```python
from build123d import *

# Parameters (mm, degrees)
F0_R     = 22.365
F1_DEPTH = 2
F2_R     = 2.5
F3_DEPTH = 45
F4_R     = 2


# Not quite as in the source:
# - a feature of the source that left no trace in its solid (it failed there, or was rolled back) is left out


with BuildPart() as f1:
    # F0 (on Top) → F1 (new body)
    with BuildSketch(Plane.XY):
        Polygon((26.865, -15.5105149818), (26.865, 15.5105149818), (0, 31.0210299636), (-26.865, 15.5105149818), (-26.865, -15.5105149818), (0, -31.0210299636), align=None)
        Circle(F0_R, mode=Mode.SUBTRACT)
        Circle(F0_R)
    extrude(amount=F1_DEPTH)

    # F2 (on face) → F3 (join)
    with BuildSketch(Plane.XY.offset(2)):
        with Locations((-14.5547939909, 0)):
            Circle(F2_R)
        with Locations((6.3876030045, 12.604821343)):
            Circle(F2_R)
        with Locations((6.8325, -11.8342371427)):
            Circle(F2_R)
    extrude(amount=F3_DEPTH)

    # F4
    f4_edges = [f1.edges().sort_by_distance(p)[0] for p in [
        (-17.054794, 0, 47),
        (4.3325, -11.834237, 47),
        (3.887603, 12.604821, 47),
    ]]
    fillet(f4_edges, radius=F4_R)


solid = f1.part
```
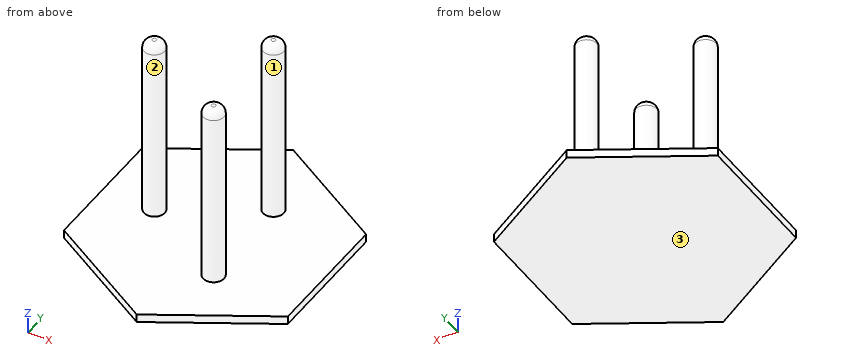
Geometry: final body of the model. Coordinates: model frame, mm. Face numbers are marked on the shaded views. Round coordinates to 2 decimals unless told otherwise and drop trailing zeros. Loops run counter-clockwise (first coordinate to the right, second up) from the corner with the lowest first, then second, coordinate; pieces in that order, holes last.
Item 1: Mould query, pull axis Y, two halves, no side actions, for the marked faces 1, 2 and 3. Classes: released by +Y, released by -Y, zero draft, split by the parting line, or undercut.
Checked values:
face 1: undercut
face 2: split by the parting line
face 3: zero draft
Item 2: Section A-A, the plane y = -5. Output: boundary loops of the cut face in (x, z) (3 decimals).
Checked values:
outline: (-26.865, 0) - (26.865, 0) - (26.865, 2) - (-26.865, 2) - close
Item 3: Contact query for flat-ended pins moving along their axis: P1, Ø2, axis at x = 1, z = 21.5, coming from the +Y side; P2, Ø1, axis at x = -10.5, y = -0.5, coming from the +Z side; P3, Ø5, axis at y = -13.5, z = 32.5, coming from the -X side; P4, Ø12, axis at x = 14, z = 42, coming from the -Y side. Output: stop coordinate, or through.
Checked values:
P1: passes through
P2: stops at z = 2
P3: stops at x = 4.33
P4: stops at y = -14.04
Item 4: Section B-B, the plane z = 25. Output: boundary loops of the cut face in (x, y).
Checked values:
outline: circle Ø5 at (-14.55, 0); circle Ø5 at (6.39, 12.6); circle Ø5 at (6.83, -11.83)
Item 5: Section C-C, the plane x = 20. Output: boundary loops of the cut face in (y, z).
Checked values:
outline: (-19.47, 0) - (19.47, 0) - (19.47, 2) - (-19.47, 2) - close
Item 6: Line query: L1, parallel to Z at x = 1, y = 7; L2, parallel to X at y = 12.5, z = 5; L3, parallel to Y at x = 5.5, z = 39. Output: solid intervals per line, ascending.
Checked values:
L1: z = 0 to 2
L2: x = 3.89 to 8.89
L3: y = -13.95 to -9.72, 10.27 to 14.94
